CAD build for the part. Positions are in the model's coordinates, mm. Face numbers are marked on the shaded views. A direction names the side the tool comes from. Coordinates: 2 decimals unless noted, no trailing zeros. Loops run counter-clockwise (first coordinate to the right, second up) from the corner with the lowest first, then second, coordinate; pieces in that order, holes last.
1) Pin check, flat tips, straight feed: pin 1 Ø6 at (x, y) = (1, 4.5) entering from +Z; pin 2 Ø1 at (x, z) = (5.5, 1.5) entering from -Y; pin 3 Ø8 at (x, z) = (-10, -4) entering from +Y. Stop position of each tip, or through.
2) Which spindle directions (+Z, -Z, +X, -X, +Y, -Y) get a long thin tool onto all of the face, cutting with end or side? Do the marked faces 1, 2 and 3. Say none if no direction does.
3) Wall check: line 1 along X through (y, z) = (-2.5, -6.25); line 2 along Y through (x, z) = (2, 0.25); line 3 along Z through (x, y) = (8, 0.25). Give the ranges that are in metal, low to high.
4) Saw through at C-C, the plane x = 8.75. Write the cut outline in (y, z).
5) Saw through at D-D, the plane y = 5. Write the cut outline in (x, z), and give its area (4 significant figures).
```python
from build123d import *

# Parameters (mm, degrees)
F2_SIZE2 = 0.5
F2_SIZE  = 0.5


with BuildPart() as f1:
    # F0 (on Front) → F1 (revolve)
    with BuildSketch(Plane.XZ):
        Polygon((15, 0), (-15, 0), (-15, -4), (-13.3, -4), (-13.3, -3), (-12.3, -3), (-12.3, -4), (-7.5, -4), (-7.5, -9), (7.5, -9), (7.5, -4), (12.3, -4), (12.3, -3), (13.3, -3), (13.3, -4), (15, -4), align=None)
    revolve(axis=Axis((-12.237907, 0, 0), (-1, 0, 0)))

    # F2
    f2_edges = [f1.edges().sort_by_distance(p)[0] for p in [
        (15, 0, 4),
        (-15, 0, 4),
    ]]
    chamfer(f2_edges, length=F2_SIZE, length2=F2_SIZE2)


solid = f1.part
```
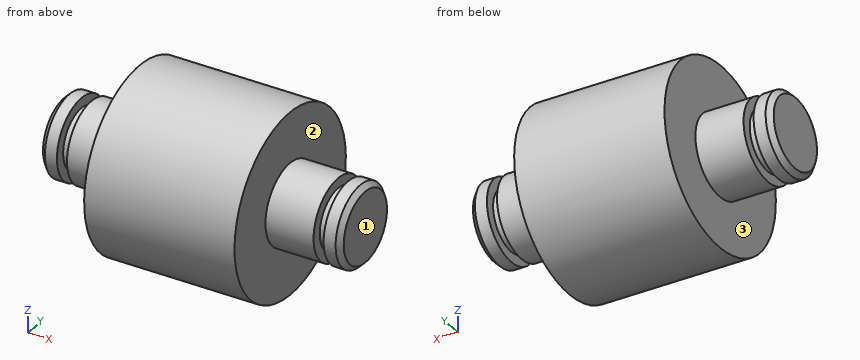
Data:
1. pin 1: stops at z = 8.87
1. pin 2: stops at y = -8.94
1. pin 3: stops at y = 8.96
2. face 1: +Z, -Z, +X, +Y, -Y
2. face 2: +X
2. face 3: -X
3. line 1: x = -7.5 to 7.5
3. line 2: y = -9 to 9
3. line 3: z = -3.99 to 3.99
4. outline: circle Ø8 at (0, 0)
5. outline: (-7.5, -7.48) - (7.5, -7.48) - (7.5, 7.48) - (-7.5, 7.48) - close
5. area: 224.5 mm2
